```python
from build123d import *

# Parameters (mm, degrees)
ESQUISSE1_R        = 1.05
BOSS_EXTRU_1_DEPTH = 1.5
CONG_1_R           = 1.5
CONG_2_R           = 1.5
ESQUISSE3_W        = 2.5
ESQUISSE3_H        = 2.5
BOSS_EXTRU_2_DEPTH = 2


with BuildPart() as part:
    # Esquisse1 → Boss.-Extru.1 (new body)
    with BuildSketch(Plane.XY):
        Polygon((-8.952173913, 8.212533242), (23.287826087, 8.212533242), (23.287826087, 5.301553174), (19.32314664, -5.987466758), (-8.952173913, -5.987466758), align=None)
        with Locations((-5.952173913, -4.387466758)):
            Circle(ESQUISSE1_R, mode=Mode.SUBTRACT)
        with Locations((-5.952173913, 6.612533242)):
            Circle(ESQUISSE1_R, mode=Mode.SUBTRACT)
        with Locations((21.687826087, 5.612533242)):
            Circle(ESQUISSE1_R, mode=Mode.SUBTRACT)
    extrude(amount=BOSS_EXTRU_1_DEPTH)

    # Congé1
    cong_1_edges = [part.edges().sort_by_distance(p)[0] for p in [
        (23.287826087, 8.212533242, 0.75),
    ]]
    fillet(cong_1_edges, radius=CONG_1_R)

    # Congé2
    cong_2_edges = [part.edges().sort_by_distance(p)[0] for p in [
        (-8.952173913, 8.212533242, 0.75),
        (19.32314664, -5.987466758, 0.75),
        (-8.952173913, -5.987466758, 0.75),
    ]]
    fillet(cong_2_edges, radius=CONG_2_R)

    # Esquisse3 → Boss.-Extru.2 (add)
    with BuildSketch(Plane(origin=(0, 0, 0), x_dir=(-1, 0, 0), z_dir=(0, 0, -1))):
        with Locations((-3.957826087, 1.112533242)):
            Rectangle(ESQUISSE3_W, ESQUISSE3_H)
    extrude(amount=BOSS_EXTRU_2_DEPTH)


solid = part.part
```
Work out the finished part from the listing and answer in its coordinate system (mm). A direction names the side the tool comes from. Give positions to 0.01 mm unless a question says otherwise; leave off trailing zeros. Order: outer loops, then holes, each group sorted by start corner. A loop starts at its lowest first (then second) coordinate and runs counter-clockwise, first axis right, second up. Notation, with made-up numbers: M 57,9.5 L 100,9.5 A20 ccw 100,16.5 Z; hole C -14.75,45.5 d7. An arc over 180 degrees is marked long. Return JSON: item names as keys, results as strings.
1) For a pull along X with two mould halves and no side action, classify faces 1 (the cylindrical face through (-6.089, 7.654, 0.74)), 2 (the cylindrical face through (22.658, 5.21, 0.74)), 3 (the flat face through (7, 1, 0)), 4 (the cylindrical face through (19.117, -5.719, 0.76)) as +X half, -X half, draft (parallel to the pull), parting line (faces both ways), or undercut.
Resolved:
{"face 1": "undercut", "face 2": "undercut", "face 3": "draft", "face 4": "+X half"}
2) A tool of negligible diameter and unlimited length cuts with its end or side. For faces 5 (the flat face through (4, -0.137, -1)), 6 (the flat face through (5.208, 1, -1)), 7 (the flat face through (2.708, 1, -1)), 8 (the flat face through (4, 2.363, -1)), from which of +Z, -Z, +X, -X, +Y, -Y can it reach the whole face along a straight path? Write none if from no direction.
Resolved:
{"face 5": "-Z, +X, -X, -Y", "face 6": "-Z, +X, +Y, -Y", "face 7": "-Z, -X, +Y, -Y", "face 8": "-Z, +X, -X, +Y"}
3) Section D-D, the plane x = 4 is taken. Write down the section's boundary in (y, z), plus the area to 3 significant figures.
Resolved:
{"outline": "M -5.99,0 L -0.14,0 L -0.14,-2 L 2.36,-2 L 2.36,0 L 8.21,0 L 8.21,1.5 L -5.99,1.5 Z", "area": "26.3 mm^2"}
4) Section C-C, the plane z = 0.45 is taken. Write down the section's boundary in (x, y), plus the area to 3 significant figures.
Resolved:
{"outline": "M -8.95,-4.49 A1.5 ccw -7.45,-5.99 L 18.26,-5.99 A1.5 ccw 19.68,-4.98 L 23.29,5.3 L 23.29,6.71 A1.5 ccw 21.79,8.21 L -7.45,8.21 A1.5 ccw -8.95,6.71 Z; hole C -5.95,-4.39 d2.1; hole C -5.95,6.61 d2.1; hole C 21.69,5.61 d2.1", "area": "423 mm^2"}
5) Each of these flat-tipped pins is pushed along its axis until it touches: pin 1 (2 mm diameter, centred on y = 1.5, z = -0.5, fed in from +X); pin 2 (1.5 mm diameter, centred on x = 6.5, y = 4.5, fed in from -Z); pin 3 (1.6 mm diameter, centred on y = 0.5, z = -1.5, fed in from -X). Where does it stop, or does it pass through?
Resolved:
{"pin 1": "x = 22.26", "pin 2": "z = 0", "pin 3": "x = 2.71"}
6) Section B-B, the plane x = 21 is taken. Write down the section's boundary in (y, z), plus the area to 3 significant figures.
Resolved:
{"outline": "M -1.21,0 L 4.82,0 L 4.82,1.5 L -1.21,1.5 Z; M 6.41,0 L 8.21,0 L 8.21,1.5 L 6.41,1.5 Z", "area": "11.8 mm^2"}
7) Section A-A, the plane y = 7 is taken. Write down the section's boundary in (x, z).
Resolved:
{"outline": "M -8.92,0 L -6.93,0 L -6.93,1.5 L -8.92,1.5 Z; M -4.98,0 L 23.26,0 L 23.26,1.5 L -4.98,1.5 Z"}
8) Straight lines are drawn through the part: line 1 along Y through (x, z) = (-5, 0.9); line 2 along Y through (x, z) = (4.5, -1.8); line 3 along Z through (x, y) = (-2.5, -2.75). For each, find the intervals that lie inside material, in ascending order. Write a range as [from, to].
Resolved:
{"line 1": "[-5.99, -4.83], [-3.94, 6.17], [7.06, 8.21]", "line 2": "[-0.14, 2.36]", "line 3": "[0, 1.5]"}
